Geometry: see drawing. Coordinates: mm, zero at the bounding-box minimum. A direction names the side the tool comes from. Coordinates: 2 decimals unless noted, no trailing zeros. Loops run counter-clockwise (first coordinate to the right, second up) from the corner with the lowest first, then second, coordinate; pieces in that order, holes last. Notation, with made-up numbers: (14, 50.25) -> (38, 50.25) arc R27 ccw to (38, 70.25) -> close; hole circle Ø6 at (72, -33). An arc over 180 degrees is marked (long way). Put each result on its own line as item: value. Start each with the question number.
1) Material intervals for L1, parallel to X at y = 0.7, z = 2.5; L2, parallel to Z at x = 36.5, y = 0.5; L3, parallel to Y at x = 34.5, z = 4.5, sorted ascending.
2) Set-up query: the marked faces 4, 5 and 6. Return all of +Z, -Z, +X, -X, +Y, -Y with unobstructed straight access to the full face (end or side cutting, diameter ignored); none if empty.
3) Cut plane A-A (y = 3.4). Return the cut outline in (x, z).
4) Cut plane C-C (z = 2.5). Return the cut outline in (x, y), plus the area to 3 significant figures.
5) Cut plane B-B (x = 36.5). Return the cut outline in (y, z).
6) Contact query for flat-ended pins moving along their axis: P1, Ø1, axis at y = 3.5, z = 11, coming from the +X side; P2, Ø1.5, axis at x = 17.5, y = 2.5, coming from the -Z side; P3, Ø6, axis at x = 23, z = 11.5, coming from the +Y side; P4, Ø0.9, axis at x = 3, y = 2, coming from the +Z side. Output: stop coordinate, or through.
7) Pull-direction query (X, two-part tool) for the marked faces 1, 2 and 3; classes: pulls with the +X half, pulls with the -X half, needs draft (parallel to the pull), parting line crosses it, or undercut.
8) Cut plane D-D (x = 3). Return the cut outline in (y, z), plus the area to 3 significant figures.
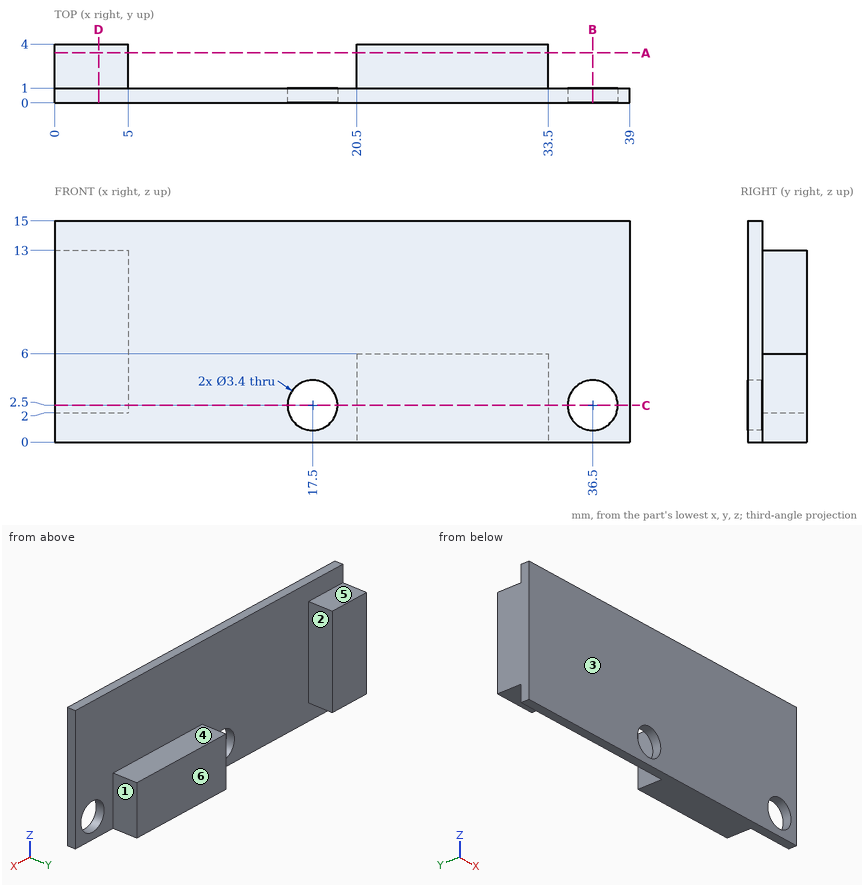
Results found:
1. L1: x = 0 to 15.8, 19.2 to 34.8, 38.2 to 39
1. L2: z = 0 to 0.8, 4.2 to 15
1. L3: y = 0 to 1
2. face 4: +Z, +X, +Y
2. face 5: +Z, +X, -X, +Y
2. face 6: +Z, -Z, +X, -X, +Y
3. outline: (0, 2) -> (5, 2) -> (5, 13) -> (0, 13) -> close; (20.5, 0) -> (33.5, 0) -> (33.5, 6) -> (20.5, 6) -> close
4. outline: (0, 0) -> (15.8, 0) -> (15.8, 1) -> (5, 1) -> (5, 4) -> (0, 4) -> close; (19.2, 0) -> (34.8, 0) -> (34.8, 1) -> (33.5, 1) -> (33.5, 4) -> (20.5, 4) -> (20.5, 1) -> (19.2, 1) -> close; (38.2, 0) -> (39, 0) -> (39, 1) -> (38.2, 1) -> close
4. area: 86.2 mm2
5. outline: (0, 0) -> (1, 0) -> (1, 0.8) -> (0, 0.8) -> close; (0, 4.2) -> (1, 4.2) -> (1, 15) -> (0, 15) -> close
6. P1: stops at x = 5
6. P2: passes through
6. P3: stops at y = 1
6. P4: stops at z = 13
7. face 1: pulls with the +X half
7. face 2: undercut
7. face 3: needs draft
8. outline: (0, 0) -> (1, 0) -> (1, 2) -> (4, 2) -> (4, 13) -> (1, 13) -> (1, 15) -> (0, 15) -> close
8. area: 48.0 mm2
